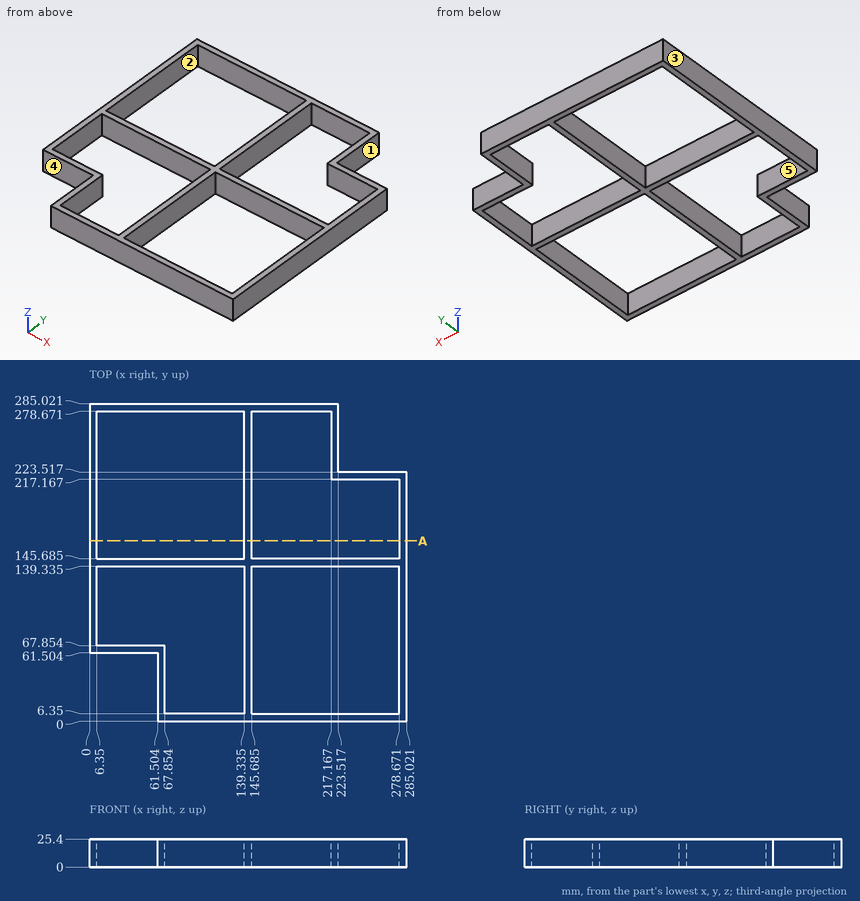
Here's the drawing with two shaded views (mm, measured from the low corner). I have some questions. A direction names the side the tool comes from. Round coordinates to 2 decimals unless told otherwise and drop trailing zeros. Use CSV: the item, a comma, the result in double quotes.
Item 1: For the marked faces 1 and 2, which set-ups out of +Z, -Z, +X, -X, +Y, -Y let a thin tool reach every point of the face, with its end or its side?
Here are the results:
face 1,"+Z, -Z, +X, +Y"
face 2,"+Z, -Z"
Item 2: If we section it at A-A on y = 162: Count the separate pieces of the cut face and the enclosed holes in it, then the cut area to 3 significant figures.
Here are the results:
separate pieces,"3"
enclosed holes,"0"
area,"484 mm²"
Item 3: I need wall thicknesses on L1, parallel to Y at x = 26.5, z = 3.75 (1 decimal). Which ranges of the line are inside material? Lowest first, please. Write a range as [from, to].
Here are the results:
L1,"y = [61.5, 67.9], [139.3, 145.7], [278.7, 285]"
Item 4: If we mould it in two halves opening along Y, with no side actions, what happens to the marked faces 3, 4 and 5? For each: pulls with the +Y half, pulls with the -Y half, needs draft (parallel to the pull), parting line crosses it, or undercut.
Here are the results:
face 3,"needs draft"
face 4,"pulls with the -Y half"
face 5,"undercut"
Item 5: Will this pin go through, and if not, where does the flat tip stop? pin 1 (7.5 mm diameter, centred on y = 260.5, z = 7.5, fed in from +X).
Here are the results:
pin 1,"stops at x = 223.52"
